```python
from build123d import *

# Parameters (mm, degrees)
SKETCH_1_R               = 1.6
EXTRUDE_1_DEPTH          = 2
SKETCH_2_R               = 61
CUT_EXTRUDE_3_DEPTH      = 0.6
SKETCH_3_R               = 3.15
CUT_EXTRUDE_4_DEPTH      = 2
CUT_EXTRUDE_6_DEPTH      = 56
CUT_EXTRUDE_6_DEPTH_BACK = 58


with BuildPart() as part:
    # Эскиз1 → Бобышка-Вытянуть1 (new body)
    with BuildSketch(Plane(origin=(0, 0, 0), x_dir=(1, 0, 0), z_dir=(0, 1, 0))):
        with BuildLine():
            ThreePointArc((-44.194173824, 48.436814511), (-48.387717364, 48.484800745), (-48.531650935, 44.293453322))
            Line((-48.531650935, 44.293453322), (-48.337535014, 44.0993374))
            Line((-48.337535014, 44.0993374), (-46.262438284, 42.024240671))
            ThreePointArc((-46.262438284, 42.024240671), (-62.49999998, 0.001572675), (-46.264553121, -42.021912433))
            Line((-46.264553121, -42.021912433), (-48.436814511, -44.194173824))
            ThreePointArc((-48.436814511, -44.194173824), (-48.484800745, -48.387717364), (-44.293453322, -48.531650935))
            Line((-44.293453322, -48.531650935), (-44.0993374, -48.337535014))
            Line((-44.0993374, -48.337535014), (-42.024240671, -46.262438284))
            ThreePointArc((-42.024240671, -46.262438284), (-0.001572675, -62.49999998), (42.021912433, -46.264553121))
            Line((42.021912433, -46.264553121), (44.194173824, -48.436814511))
            ThreePointArc((44.194173824, -48.436814511), (48.387717364, -48.484800745), (48.531650935, -44.293453322))
            Line((48.531650935, -44.293453322), (48.337535014, -44.0993374))
            Line((48.337535014, -44.0993374), (46.262438284, -42.024240671))
            ThreePointArc((46.262438284, -42.024240671), (62.49999998, -0.001572675), (46.264553121, 42.021912433))
            Line((46.264553121, 42.021912433), (48.436814511, 44.194173824))
            ThreePointArc((48.436814511, 44.194173824), (48.484800745, 48.387717364), (44.293453322, 48.531650935))
            Line((44.293453322, 48.531650935), (44.0993374, 48.337535014))
            Line((44.0993374, 48.337535014), (42.024240671, 46.262438284))
            ThreePointArc((42.024240671, 46.262438284), (0.001572675, 62.49999998), (-42.021912433, 46.264553121))
            Line((-42.021912433, 46.264553121), (-44.194173824, 48.436814511))
        make_face()
        with Locations(Location((-46.315494168, -46.315494168, 0), (0, 0, 270))):
            Circle(SKETCH_1_R, mode=Mode.SUBTRACT)
        with Locations(Location((46.315494168, -46.315494168, 0), (0, 0, 270))):
            Circle(SKETCH_1_R, mode=Mode.SUBTRACT)
        with Locations(Location((-46.315494168, 46.315494168, 0), (0, 0, 270))):
            Circle(SKETCH_1_R, mode=Mode.SUBTRACT)
        with Locations(Location((46.315494168, 46.315494168, 0), (0, 0, 270))):
            Circle(SKETCH_1_R, mode=Mode.SUBTRACT)
    extrude(amount=EXTRUDE_1_DEPTH)

    # Эскиз2 → Вырез-Вытянуть3 (cut)
    with BuildSketch(Plane(origin=(0, 2, 0), x_dir=(1, 0, 0), z_dir=(0, 1, 0))):
        with Locations(Location((0, 0, 0), (0, 0, 270))):
            Circle(SKETCH_2_R)
    extrude(amount=-CUT_EXTRUDE_3_DEPTH, mode=Mode.SUBTRACT)

    # Эскиз3 → Вырез-Вытянуть4 (cut)
    with BuildSketch(Plane(origin=(0, 1.4, 0), x_dir=(1, 0, 0), z_dir=(0, 1, 0))):
        with Locations(Location((0, 0, 0), (0, 0, 270))):
            Circle(SKETCH_3_R)
    extrude(amount=-CUT_EXTRUDE_4_DEPTH, mode=Mode.SUBTRACT)

    # Эскиз6 → Вырез-Вытянуть6 (cut, two sides: drawn at the far end of the back side and taken through both)
    with BuildSketch(Plane(origin=(0, 0, 0), x_dir=(1, 0, 0), z_dir=(0, 1, 0)).offset(-CUT_EXTRUDE_6_DEPTH_BACK)):
        Polygon((-21.818311129, -55.668605856), (-8.341675093, -22.760328818), (-1, -24.220678791), (-1, -59.783022844), align=None)
    extrude(amount=CUT_EXTRUDE_6_DEPTH + CUT_EXTRUDE_6_DEPTH_BACK, mode=Mode.SUBTRACT)


solid = part.part
```
The model under review builds one solid part; all positions refer to its coordinate system, in mm. A direction names the side the tool comes from. Give positions to 0.01 mm unless a question says otherwise; leave off trailing zeros. Write each loop counter-clockwise with the first axis right and the second up, starting at its lowest first coordinate (ties: lowest second). Pieces come first, ordered by that corner, then holes. Notation, with made-up numbers: M 44.25,87.25 L 87.25,87.25 A22 cw 87.25,100.25 Z; hole C 70,13 d1. An arc over 180 degrees is marked long. Write item = value, one per line. Start each with the question number.
Q1. We need section A-A (z = 0). State the section outline as (x, y) points, plus the area to 3 significant figures.
Q2. We need section D-D (z = -15). State the section outline as (x, y) points, plus the area to 3 significant figures.
Q3. We need section C-C (x = 19). State the section outline as (y, z) points.
Q4. For line 1 (Z direction, x = -42, y = 1.9); line 2 (Y direction, x = 8, z = -4); line 3 (Z direction, x = -49, y = 0.35), list the stretches that pass through material, from the lowest coordinate up.
Q5. We need section B-B (y = 0.85). State the section outline as (x, z) points.
Q6. Clearance check with flat-ended pins moving along their axes: pin 1 (4 mm diameter, centred on x = -15, z = 29, fed in from +Y); pin 2 (1.1 mm diameter, centred on y = 0.5, z = 47, fed in from -X); pin 3 (1 mm diameter, centred on x = 46.5, z = 32.5, fed in from -Y); pin 4 (1 mm diameter, centred on x = -15, y = 0.5, fed in from -Z). State where each tip first meets the part, or that it passes through.
Q7. Mouldability with a two-part tool opening along X and no side actions: class faces 1 (the face through (45.342, 0.986, -47.585)), 2 (the face through (62.497, 0.986, 0.647)), 3 (the face through (-62.497, 0.986, -0.647)), 4 (the face through (-15.174, 0.69, 39.445)) as released by +X, released by -X, zero draft, split by the parting line, or undercut.
Q8. Machinability: for faces 5 (the face through (-11.263, 0.69, 57.755)), 6 (the face through (-0.647, 0.986, 62.497)), 7 (the face through (-13, 1.4, -1)), which of the approach directions +Z, -Z, +X, -X, +Y, -Y give a long, thin tool a straight path to every point of the face, cutting with its end or side? Answer none if there is none.
Result set:
q1.outline = M -62.5,0 L -3.15,0 L -3.15,1.4 L -61,1.4 L -61,2 L -62.5,2 Z; M 3.15,0 L 62.5,0 L 62.5,2 L 61,2 L 61,1.4 L 3.15,1.4 Z
q1.area = 168 mm2
q2.outline = M -60.67,0 L 60.67,0 L 60.67,2 L 59.13,2 L 59.13,1.4 L -59.13,1.4 L -59.13,2 L -60.67,2 Z
q2.area = 172 mm2
q3.outline = M 0,-59.54 L 2,-59.54 L 2,-57.97 L 1.4,-57.97 L 1.4,57.97 L 2,57.97 L 2,59.54 L 0,59.54 Z
q4.line_1 = -46.28 to -44.24, 44.24 to 46.28
q4.line_2 = 0 to 1.4
q4.line_3 = -47.65 to -44.98, -38.8 to 38.8, 44.98 to 47.65
q5.outline = M -48.53,-44.29 A3 ccw -44.19,-48.44 L -42.02,-46.26 A62.5 ccw 42.02,-46.26 L 44.29,-48.53 A3 ccw 48.44,-44.19 L 46.26,-42.02 A62.5 ccw 46.26,42.02 L 48.53,44.29 A3 ccw 44.19,48.44 L 42.02,46.26 A62.5 ccw -42.02,46.26 L -44.29,48.53 A3 ccw -48.44,44.19 L -46.26,42.02 A62.5 ccw -46.26,-42.02 Z; hole C -46.32,-46.32 d3.2; hole C -46.32,46.32 d3.2; hole M -21.82,55.67 L -8.34,22.76 L -1,24.22 L -1,59.78 Z; hole C 0,0 d6.3; hole C 46.32,-46.32 d3.2; hole C 46.32,46.32 d3.2
q6.pin_1 = 1.4
q6.pin_2 = -49.31
q6.pin_3 = 0
q6.pin_4 = -60.79
q7.face_1 = undercut
q7.face_2 = released by +X
q7.face_3 = released by -X
q7.face_4 = undercut
q8.face_5 = +Y, -Y
q8.face_6 = +Z, +Y, -Y
q8.face_7 = +Y
